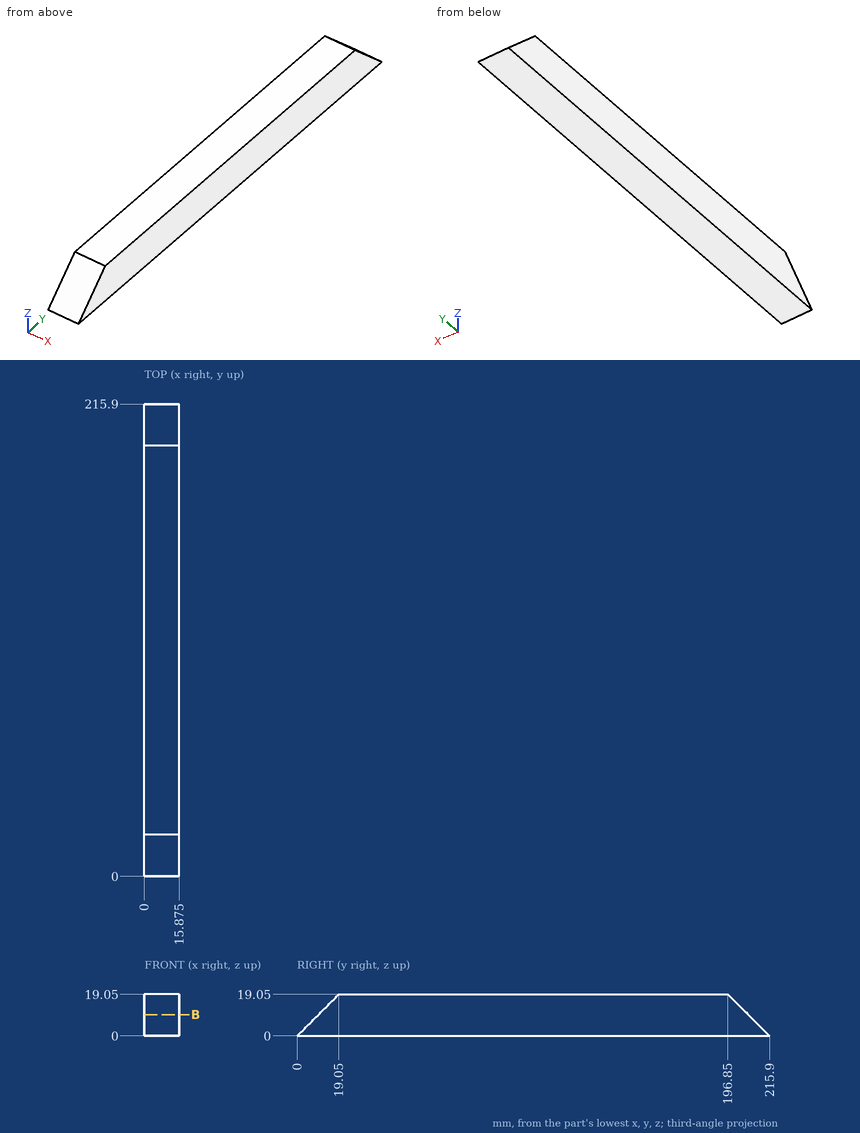
The drawing under review shows one solid part. Ordinate dimensions are in mm from its lowest x, y, z. Coordinates: 2 decimals unless noted, no trailing zeros. Write each loop counter-clockwise with the first axis right and the second up, starting at its lowest first coordinate (ties: lowest second). Pieces come first, ordered by that corner, then holes. Notation, with made-up numbers: M -6,-38.5 L 28,-38.5 A15 cw 28,-25.5 Z; hole C -38.75,-8.5 d5. An arc over 180 degrees is marked long. Put each result on its own line as item: value.
1) Wall thickness on probe 1 along Y at (x, z) = (8, 12.5); probe 2 along Z at (x, y) = (6, 198.5); probe 3 along Z at (x, y) = (5.25, 202.5): over which ranges is each line inside the solid? List them lowest first. Write a range as [from, to].
Computed:
probe 1: y = [12.5, 203.4]
probe 2: z = [0, 17.4]
probe 3: z = [0, 13.4]
2) Clearance check with flat-ended pins moving along their axes: pin 1 Ø2 at (x, z) = (5.5, 11) entering from -Y; pin 2 Ø8 at (x, z) = (3.5, 9) entering from -Y; pin 3 Ø3 at (x, z) = (4, 10) entering from +Y. State where each tip first meets the part, or that it passes through.
Computed:
pin 1: stops at y = 10
pin 2: stops at y = 5
pin 3: stops at y = 207.4
3) Add section B-B on z = 9.75. Give the boundary of the cut face in (x, y) (3 decimals), then the cut area to 3 significant figures.
Computed:
outline: M 0,9.75 L 15.875,9.75 L 15.875,206.15 L 0,206.15 Z
area: 3,120 mm2
